```python
from build123d import *

# Parameters (mm, degrees)
F0_R     = 2.6468200674
F0_R_2   = 2.4751284116
F1_DEPTH = 23.0632
F3_D     = 19.05
F3_DEPTH = 15.24
F3_TIP   = 5.7231973962
F5_D     = 15.748
F5_DEPTH = 17.78
F5_TIP   = 4.7311765142
F6_DEPTH = 76.2
F7_D     = 15.748
F7_DEPTH = 78.74
F7_TIP   = 4.7311765142


with BuildPart() as f1:
    # F0 (on Front) → F1 (new body)
    with BuildSketch(Plane.XZ):
        with BuildLine():
            ThreePointArc((-13.3964658612, 6.7509404916), (-11.4760473771, 4.8729949891), (-8.8789812826, 4.1874775452))
            Line((-8.8789812826, 4.1874775452), (10.0976222454, 4.1874775452))
            Line((10.0976222454, 4.1874775452), (10.4250187174, 4.1874775452))
            ThreePointArc((10.4250187174, 4.1874775452), (14.1459697805, 5.7287459405), (15.6872381758, 9.4496970036))
            Line((15.6872381758, 9.4496970036), (15.6872381758, 25.9596970036))
            ThreePointArc((15.6872381758, 25.9596970036), (16.0113150838, 27.7778559021), (16.9436288703, 29.3720700112))
            Line((16.9436288703, 29.3720700112), (17.6345340249, 30.1831324991))
            ThreePointArc((17.6345340249, 30.1831324991), (18.8853795407, 33.8370197817), (17.3047602431, 37.3608173659))
            Line((17.3047602431, 37.3608173659), (13.7047539976, 40.875485311))
            ThreePointArc((13.7047539976, 40.875485311), (12.0132715508, 41.9838194669), (10.0286990154, 42.3723929102))
            Line((10.0286990154, 42.3723929102), (1.3647818566, 42.3723929102))
            ThreePointArc((1.3647818566, 42.3723929102), (-1.1423679176, 41.7367438487), (-3.0438160811, 39.9833629429))
            Line((-3.0438160811, 39.9833629429), (-15.6918746521, 20.5762875984))
            Line((-15.6918746521, 20.5762875984), (-15.6918746521, 10.5932559313))
            Line((-15.6918746521, 10.5932559313), (-13.3964658612, 6.7509404916))
        make_face()
        with Locations((-8.8789812826, 9.4496970036)):
            Circle(F0_R, mode=Mode.SUBTRACT)
        with Locations((10.0286990154, 37.1101734518)):
            Circle(F0_R_2, mode=Mode.SUBTRACT)
    extrude(amount=F1_DEPTH)

    # F3
    with Locations(Plane.XZ.offset(23.0632)):
        with Locations((0.6101487425, 21.472733464)):
            Hole(F3_D / 2, depth=F3_DEPTH)
            with Locations((0, 0, -(F3_DEPTH + F3_TIP / 2))):  # 118° drill point
                Cone(0, F3_D / 2, F3_TIP, mode=Mode.SUBTRACT)

    # F5
    with Locations(Plane(origin=(0, 0, 4.1874775452), x_dir=(1, 0, 0), z_dir=(0, 0, -1))):
        with Locations((0.7486785246, 11.6532988795)):
            Hole(F5_D / 2, depth=F5_DEPTH)
            with Locations((0, 0, -(F5_DEPTH + F5_TIP / 2))):  # 118° drill point
                Cone(0, F5_D / 2, F5_TIP, mode=Mode.SUBTRACT)

    # F4 (on face) → F6 (join)
    with BuildSketch(Plane(origin=(0, 0, 4.1874775452), x_dir=(1, 0, 0), z_dir=(0, 0, -1))):
        with BuildLine():
            ThreePointArc((9.8926785246, 11.6532988795), (-5.4467560676, 18.3785740571), (0, 2.54))
            ThreePointArc((0, 2.54), (6.9441131167, 4.9280237019), (9.8926785246, 11.6532988795))
        make_face()
    extrude(amount=F6_DEPTH)

    # F7 (one way)
    with BuildSketch(Plane.XY.offset(4.1874775452)):
        with Locations((0.7486785246, -11.6532988795)):
            Circle(F7_D / 2)
    extrude(amount=-F7_DEPTH, mode=Mode.SUBTRACT)
    with Locations(Plane.XY.offset(4.1874775452)):
        with Locations((0.7486785246, -11.6532988795)):
            with Locations((0, 0, -(F7_DEPTH + F7_TIP / 2))):  # 118° drill point
                Cone(0, F7_D / 2, F7_TIP, mode=Mode.SUBTRACT)


solid = f1.part
```
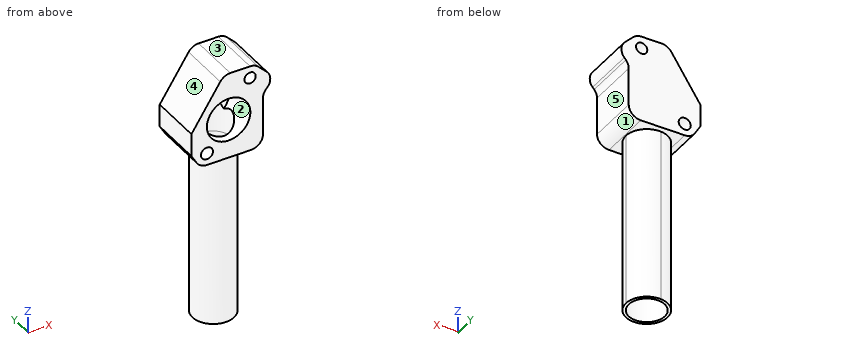
Model file for the job. Use its own axes, mm. Face numbers are marked on the shaded views. A direction names the side the tool comes from. Coordinates: 2 decimals unless noted, no trailing zeros. Order: outer loops, then holes, each group sorted by start corner. A loop starts at its lowest first (then second) coordinate and runs counter-clockwise, first axis right, second up. Notation, with made-up numbers: (82.5, 71) -> (108.5, 71) arc R15 cw to (108.5, 89) -> close; hole circle Ø8 at (29.25, -18). An arc over 180 degrees is marked (long way). Return JSON: item names as keys, results as strings.
Item 1: Wall check: line 1 along Y through (x, z) = (1, -55); line 2 along Z through (x, y) = (-7.5, -16.25); line 3 along X through (y, z) = (-6.75, 7.5). Give the ranges that are in metal, low to high. Write a range as from..to.
Model answer:
{"line 1": "y = -20.79..-19.52, -3.78..-2.51", "line 2": "z = 4.19..7.19, 11.71..16.48, 26.47..33.15", "line 3": "x = -13.84..-10.67, -7.09..-5.41, 6.91..15.31"}
Item 2: Mould opens along X. For the marked faces 1, 2 and 3 say: pulls with the +X half, pulls with the -X half, needs draft (parallel to the pull), parting line crosses it, or undercut.
Model answer:
{"face 1": "pulls with the +X half", "face 2": "undercut", "face 3": "needs draft"}
Item 3: Slice it at B-B (z = -25.5). Write the cut outline in (x, y).
Model answer:
{"outline": "circle Ø18.29 at (0.75, -11.65); hole circle Ø15.75 at (0.75, -11.65)"}
Item 4: Pin check, flat tips, straight feed: P1, Ø12, axis at x = -1, y = -10.5, coming from the -Z side; P2, Ø3, axis at x = -4.5, y = -8, coming from the +Z side; P3, Ø1.5, axis at y = -7.5, z = -26.5, coming from the +X side; P4, Ø8, axis at x = 1.5, z = -20, coming from the +Y side. Stop position of each tip, or through.
Model answer:
{"P1": "stops at z = -72.01", "P2": "stops at z = 40.05", "P3": "stops at x = 9.24", "P4": "stops at y = -2.51"}
Item 5: 3-axis set-ups, long thin cutter, end or side, ignore diameter. For the marked faces 4 and 5: which of +Z, -Z, +X, -X, +Y, -Y reach the whole face in a straight line?
Model answer:
{"face 4": "+Z, -X, +Y, -Y", "face 5": "-Z, +X, +Y, -Y"}
